The listing builds one solid part. Answer for the finished solid, in the listing's coordinates (mm). A direction names the side the tool comes from. Round coordinates to 2 decimals unless told otherwise and drop trailing zeros. Loops run counter-clockwise (first coordinate to the right, second up) from the corner with the lowest first, then second, coordinate; pieces in that order, holes last. Notation, with made-up numbers: (23.5, 64) -> (69.5, 64) arc R9 cw to (69.5, 78) -> close; hole circle Ø3 at (30, 50). An arc over 180 degrees is marked (long way). Use a Markdown table: item, result. Add a question column.
Q1. Section A-A on z = 0 is taken. Give the vertices of the cut face in (x, y), then the cut area to 3 significant figures.
Q2. Section B-B on x = 60.5 is taken. Give the vertices of the cut face in (y, z), then the cut area to 3 significant figures.
Q3. Section C-C on y = 0 is taken. Give the vertices of the cut face in (x, z), then the cut area to 3 significant figures.
Q4. Given pin 1 Ø12.5 at (x, z) = (0, 0) entering from +Y; pin 2 Ø3 at (y, z) = (-5.5, 3) entering from -X; pin 3 Ø6 at (y, z) = (0, 0) entering from +X, each flat-ended and moving along its own axis, determine where each tip first touches the part or whether it passes through.
Q5. Consider line 1 (Z direction, x = 0, y = 11); line 2 (X direction, y = 9.75, z = 0); line 3 (Y direction, x = 58.5, z = 0). Determine where each line is inside the solid, lowest interval first.
Q6. Which of the six approach directions +Z, -Z, +X, -X, +Y, -Y give full straight-line access (tool end or side, diameter ignored) to faces 1 (the flat face through (65, 3, 3)), 2 (the flat face through (-4, -5, -3)), 3 (the cylindrical face through (59.93, 3.67, -0.81))?
Q7. For a pull along X with two mould halves and no side action, classify faces 4 (the flat face through (55, 0, 0)), 5 (the cylindrical face through (-2.9, 8.7, -3.78)), 6 (the cylindrical face through (-10.76, 8.7, 0.24)) as released by +X, released by -X, zero draft, split by the parting line, or undercut.
Q8. Section D-D on z = 7 is taken. Give the vertices of the cut face in (x, y).
from build123d import *

# Parameters (mm, degrees)
SKETCH2_W               = 30
SKETCH2_H               = 30
BOSS_EXTRUDE3_DEPTH     = 12.5
CUT_EXTRUDE1_DEPTH      = 25.622144504
CUT_EXTRUDE1_DEPTH_BACK = 25.622144504
SKETCH1_R               = 4.7625
CUT_EXTRUDE2_DEPTH      = 30.061583319
CUT_EXTRUDE2_DEPTH_BACK = 30.061583319
SKETCH3_W               = 10.7625
SKETCH3_H               = 10
SKETCH5_W               = 21.525
SKETCH5_H               = 25
BOSS_EXTRUDE4_DEPTH     = 50
CUT_EXTRUDE3_DEPTH      = 78.537331734
CUT_EXTRUDE3_DEPTH_BACK = 10
SKETCH6_R               = 3.7592


with BuildPart() as part:
    # Sketch2 → Boss-Extrude3 (new, symmetric)
    with BuildSketch(Plane(origin=(0, 0, 0), x_dir=(1, 0, 0), z_dir=(0, 1, 0))):
        Rectangle(SKETCH2_W, SKETCH2_H)
    extrude(amount=BOSS_EXTRUDE3_DEPTH, both=True)

    # Sketch1 → Cut-Extrude1 (cut, two sides: drawn at the far end of the back side and taken through both)
    with BuildSketch(Plane(origin=(0, 0, 0), x_dir=(1, 0, 0), z_dir=(0, 1, 0)).offset(-CUT_EXTRUDE1_DEPTH_BACK)):
        with Locations(Location((0, 0, 0), (0, 0, 270))):
            Circle(SKETCH1_R)
        with BuildLine():
            ThreePointArc((0, -10.7625), (-10.7625, 0), (0, 10.7625))
            Line((0, 10.7625), (15, 10.7625))
            Line((15, 10.7625), (15, 15))
            Line((15, 15), (-15, 15))
            Line((-15, 15), (-15, -15))
            Line((-15, -15), (15, -15))
            Line((15, -15), (15, -10.7625))
            Line((15, -10.7625), (0, -10.7625))
        make_face()
    extrude(amount=CUT_EXTRUDE1_DEPTH + CUT_EXTRUDE1_DEPTH_BACK, mode=Mode.SUBTRACT)

    # Sketch3 → Cut-Extrude2 (cut, two sides: drawn at the far end of the back side and taken through both)
    with BuildSketch(Plane.XY.offset(10.7625).offset(-CUT_EXTRUDE2_DEPTH_BACK)):
        with BuildLine():
            Line((0, -5), (5.665118464, -5))
            ThreePointArc((5.665118464, -5), (7.186330553, 0), (5.665118464, 5))
            Line((5.665118464, 5), (0, 5))
            Line((0, 5), (0, -5))
        make_face()
        with Locations((-5.38125, 0)):
            Rectangle(SKETCH3_W, SKETCH3_H)
    extrude(amount=CUT_EXTRUDE2_DEPTH + CUT_EXTRUDE2_DEPTH_BACK, mode=Mode.SUBTRACT)

    # Sketch5 → Boss-Extrude4 (add)
    with BuildSketch(Plane(origin=(15, 0, 0), x_dir=(0, 0, -1), z_dir=(1, 0, 0))):
        Rectangle(SKETCH5_W, SKETCH5_H)
    extrude(amount=BOSS_EXTRUDE4_DEPTH)

    # Sketch6 → Cut-Extrude3 (cut, two sides: drawn at the far end of the back side and taken through both)
    with BuildSketch(Plane(origin=(65, 0, 0), x_dir=(0, 0, -1), z_dir=(1, 0, 0)).offset(-CUT_EXTRUDE3_DEPTH_BACK)):
        with Locations(Location((0, 0, 0), (0, 0, 180))):
            Circle(SKETCH6_R)
    extrude(amount=CUT_EXTRUDE3_DEPTH + CUT_EXTRUDE3_DEPTH_BACK, mode=Mode.SUBTRACT)


solid = part.part
Checked values:
| question | item | result |
|---|---|---|
| 1 | outline | (-10.76, -12.5) -> (-4.76, -12.5) -> (-4.76, -5) -> (-10.76, -5) -> close; (-10.76, 5) -> (-4.76, 5) -> (-4.76, 12.5) -> (-10.76, 12.5) -> close; (4.76, -12.5) -> (65, -12.5) -> (65, -3.76) -> (55, -3.76) -> (55, 3.76) -> (65, 3.76) -> (65, 12.5) -> (4.76, 12.5) -> (4.76, 5) -> (5.67, 5) arc R8.98 cw to (5.67, -5) -> (4.76, -5) -> close |
| 1 | area | 1,500 mm2 |
| 2 | outline | (-12.5, -10.76) -> (12.5, -10.76) -> (12.5, 10.76) -> (-12.5, 10.76) -> close; hole circle Ø7.52 at (0, 0) |
| 2 | area | 494 mm2 |
| 3 | outline | (7.19, -10.76) -> (65, -10.76) -> (65, -3.76) -> (55, -3.76) -> (55, 3.76) -> (65, 3.76) -> (65, 10.76) -> (7.19, 10.76) -> close |
| 3 | area | 1,170 mm2 |
| 4 | pin 1 | stops at y = 12.5 |
| 4 | pin 2 | stops at x = -10.66 |
| 4 | pin 3 | stops at x = 55 |
| 5 | line 1 | z = -10.76 to -4.76, 4.76 to 10.76 |
| 5 | line 2 | x = -10.76 to -4.76, 4.76 to 65 |
| 5 | line 3 | y = -12.5 to -3.76, 3.76 to 12.5 |
| 6 | face 1 | +Z, -Z, +X, +Y, -Y |
| 6 | face 2 | +Z, -Z, -X |
| 6 | face 3 | +X |
| 7 | face 4 | released by +X |
| 7 | face 5 | undercut |
| 7 | face 6 | released by -X |
| 8 | outline | (-8.18, -12.5) -> (65, -12.5) -> (65, 12.5) -> (-8.18, 12.5) -> (-8.18, 5) -> (5.67, 5) arc R8.98 cw to (5.67, -5) -> (-8.18, -5) -> close |
